```python
from build123d import *

# Parameters (mm, degrees)
BASE_FLANGE1_DEPTH = 130
FILLET1_R          = 10
SKETCH6_R          = 3.5
CUT_EXTRUDE1_DEPTH = 10
SKETCH7_R          = 9
CUT_EXTRUDE2_DEPTH = 2


# Sheet-metal steps are written as plain solids
with BuildPart() as part:
    # Sketch1 → Base-Flange1 (new body)
    with BuildSketch(Plane.XY):
        with BuildLine():
            Line((0, 100), (0, 4))
            ThreePointArc((0, 4), (-1.171572875, 1.171572875), (-4, 0))
            Line((-4, 0), (-30, 0))
            Line((-30, 0), (-30, 2))
            Line((-30, 2), (-4, 2))
            ThreePointArc((-4, 2), (-2.585786438, 2.585786438), (-2, 4))
            Line((-2, 4), (-2, 100))
            Line((-2, 100), (0, 100))
        make_face()
    extrude(amount=BASE_FLANGE1_DEPTH)

    # Fillet1
    fillet1_edges = [part.edges().sort_by_distance(p)[0] for p in [
        (-1, 100, 130),
        (-1, 100, 0),
        (-30, 1, 130),
        (-30, 1, 0),
    ]]
    fillet(fillet1_edges, radius=FILLET1_R)

    # Sketch6 → Cut-Extrude1 (cut)
    with BuildSketch(Plane(origin=(0, 2, 0), x_dir=(1, 0, 0), z_dir=(0, 1, 0))):
        with Locations(Location((-15, -15, 0), (0, 0, 270))):
            Circle(SKETCH6_R)
        with Locations(Location((-15, -115, 0), (0, 0, 270))):
            Circle(SKETCH6_R)
    extrude(amount=-CUT_EXTRUDE1_DEPTH, mode=Mode.SUBTRACT)

    # Sketch7 → Cut-Extrude2 (cut)
    with BuildSketch(Plane(origin=(0, 0, 0), x_dir=(0, 0, -1), z_dir=(1, 0, 0))):
        with Locations(Location((-65, 84.499999997, 0), (0, 0, 90))):
            Circle(SKETCH7_R)
    extrude(amount=-CUT_EXTRUDE2_DEPTH, mode=Mode.SUBTRACT)


solid = part.part
```
Work out the finished part from the listing and answer in its coordinate system (mm). A direction names the side the tool comes from. Give positions to 0.01 mm unless a question says otherwise; leave off trailing zeros. Order: outer loops, then holes, each group sorted by start corner. A loop starts at its lowest first (then second) coordinate and runs counter-clockwise, first axis right, second up. Notation, with made-up numbers: (40.25, -17) - (68.25, -17) arc R25 ccw to (68.25, 20) - close; hole circle Ø8 at (-20.5, 6). An arc over 180 degrees is marked (long way). One line per item, written item: value. Start each with the question number.
1. Consider line 1 (Z direction, x = -0.9, y = 84.5); line 2 (Y direction, x = -7, z = 35); line 3 (X direction, y = 54.5, z = 32.5). Determine where each line is inside the solid, lowest interval first.
2. Section A-A, the plane y = 84.5 is taken. Write down the section's boundary in (x, z).
3. Section D-D, the plane z = 30 is taken. Write down the section's boundary in (x, y).
4. Which of the six approach directions +Z, -Z, +X, -X, +Y, -Y give full straight-line access (tool end or side, diameter ignored) to faces 5 (the face through (-17, 0, 64)), 6 (the face through (-2, 51, 64))?
5. Section B-B, the plane x = -15 is taken. Write down the section's boundary in (y, z), then the cut area to 3 significant figures.
6. Each of these flat-tipped pins is pushed along its axis until it touches: pin 1 Ø12 at (y, z) = (50.5, 58) entering from -X; pin 2 Ø4 at (x, z) = (-15.5, 49.5) entering from +Y; pin 3 Ø4 at (x, z) = (-15, 115) entering from +Y. Where does it stop, or does it pass through?
7. Section C-C, the plane z = 15 is taken. Write down the section's boundary in (x, y), then the cut area to 3 significant figures.
8. For a pull along Z with two mould halves and no side action, classify faces 1 (the face through (-16.341, 1.014, 118.233)), 2 (the face through (0, 53, 64)), 3 (the face through (-0.986, 88.653, 57.015)), 4 (the face through (-1.8, 35.2, 130)) as released by +Z, released by -Z, zero draft, split by the parting line, or undercut.
Filled sheet:
1. line 1: 0 to 56, 74 to 130
1. line 2: 0 to 2
1. line 3: -2 to 0
2. outline: (-2, 0) - (0, 0) - (0, 56) - (-2, 56) - close; (-2, 74) - (0, 74) - (0, 130) - (-2, 130) - close
3. outline: (-30, 0) - (-4, 0) arc R4 ccw to (0, 4) - (0, 100) - (-2, 100) - (-2, 4) arc R2 cw to (-4, 2) - (-30, 2) - close
4. face 5: +Z, -Z, +X, -X, -Y
4. face 6: +Z, -Z, -X, +Y
5. outline: (0, 0) - (2, 0) - (2, 11.5) - (0, 11.5) - close; (0, 18.5) - (2, 18.5) - (2, 111.5) - (0, 111.5) - close; (0, 118.5) - (2, 118.5) - (2, 130) - (0, 130) - close
5. area: 232 mm²
6. pin 1: x = -2
6. pin 2: y = 2
6. pin 3: through
7. outline: (-30, 0) - (-18.5, 0) - (-18.5, 2) - (-30, 2) - close; (-11.5, 0) - (-4, 0) arc R4 ccw to (0, 4) - (0, 100) - (-2, 100) - (-2, 4) arc R2 cw to (-4, 2) - (-11.5, 2) - close
7. area: 239 mm²
8. face 1: undercut
8. face 2: zero draft
8. face 3: undercut
8. face 4: released by +Z
